Check sheet for the modelled part. Datum: model origin and axes. Units: mm. A direction names the side the tool comes from. Give positions to 0.01 mm unless a question says otherwise; leave off trailing zeros. Write each loop counter-clockwise with the first axis right and the second up, starting at its lowest first coordinate (ties: lowest second). Pieces come first, ordered by that corner, then holes. Notation, with made-up numbers: M 72.25,81.25 L 96.25,81.25 A19 ccw 96.25,108.25 Z; hole C -15,22 d9. An arc over 180 degrees is marked long. Use CSV: the item, a comma, the result in double quotes. Start each with the question number.
1. Cross-section at D-D, the plane z = -32. Enter the section's corners in (x, y).
2. Mould release check, pull along Z, two halves, no side actions. Record for faces 4 (the face through (-21, 43, -23.55)), 5 (the face through (-21, 43, 18.45)), 6 (the face through (-21.29, 35.22, -2.83)): +Z half, -Z half, draft (parallel to the pull), parting line (faces both ways), or undercut.
3. Cross-section at C-C, the plane z = 12. Enter the section's corners in (x, y).
4. Access from +Z, -Z, +X, -X, +Y, -Y to the whole of each face (thin tool, end or side, straight path). Record for faces 1 (the face through (-21, 38, 25)), 2 (the face through (0, 24, -3)), 3 (the face through (-21, 38, -30)).
5. Depth check by flat-ended pin: P1, Ø6.5, axis at x = -15, z = 26.5, coming from the +Y side; P2, Ø3, axis at x = -25.5, y = 43, coming from the -Z side; P3, Ø1, axis at x = 9, z = 27, coming from the +Y side. Enter the tip coordinate at first touch or a pass-through.
6. Cross-section at A-A, the plane x = -12. Enter the section's corners in (y, z).
7. Scan lines: line 1 (Y direction, x = 2, z = -31); line 2 (X direction, y = 44, z = -15); line 3 (Y direction, x = -25.5, z = 18.5). Record each from-to range of solid material in increasing order.
8. Cross-section at B-B, the plane y = 5.5. Enter the section's corners in (x, z), and give its area (3 significant figures).
from build123d import *

# Parameters (mm, degrees)
BOSS_EXTRUDE1_DEPTH = 21
BOSS_EXTRUDE2_DEPTH = 14


with BuildPart() as part:
    # Sketch1 → Boss-Extrude1 (new body)
    with BuildSketch(Plane(origin=(0, 0, 0), x_dir=(0, 0, -1), z_dir=(1, 0, 0))):
        with BuildLine():
            Line((-45.865633075, 14), (-45.865633075, 0))
            Line((-45.865633075, 0), (54.134366925, 0))
            Line((54.134366925, 0), (54.134366925, 14))
            Line((54.134366925, 14), (36.550387597, 38))
            Line((36.550387597, 38), (23.550387597, 38))
            Line((23.550387597, 38), (23.550387597, 48))
            Line((23.550387597, 48), (15.333333333, 48))
            ThreePointArc((15.333333333, 48), (2.550387597, 35.217054264), (-10.23255814, 48))
            Line((-10.23255814, 48), (-18.449612403, 48))
            Line((-18.449612403, 48), (-18.449612403, 38))
            Line((-18.449612403, 38), (-31.449612403, 38))
            Line((-31.449612403, 38), (-45.865633075, 14))
        make_face()
    extrude(amount=-BOSS_EXTRUDE1_DEPTH)

    # Mirror1: part across plane


with BuildPart() as part_1:
    add(part.part)
    add(part.part.mirror(Plane.ZY.offset(21)))

    # Sketch3 → Boss-Extrude2 (add)
    with BuildSketch(Plane.XZ):
        with BuildLine():
            Line((0, 27.865633075), (0, 24.200007191))
            Line((0, 24.200007191), (0, -20.725134363))
            Line((0, -20.725134363), (0, -36.134366925))
            ThreePointArc((0, -36.134366925), (22.627416998, -26.761783923), (32, -4.134366925))
            ThreePointArc((32, -4.134366925), (22.627416998, 18.493050073), (0, 27.865633075))
        make_face()
        with BuildLine():
            Line((0, -20.725134363), (0, 24.200007191))
            Line((0, 24.200007191), (0, 27.865633075))
            ThreePointArc((0, 27.865633075), (-32, -4.134366925), (0, -36.134366925))
            Line((0, -36.134366925), (0, -20.725134363))
        make_face()
    extrude(amount=-BOSS_EXTRUDE2_DEPTH)


solid = part_1.part
Worked answers:
1,outline,"M -42,0 L 15.73,0 L 15.73,14 L 0,14 L 0,38 L -42,38 Z"
2,face 4,"-Z half"
2,face 5,"+Z half"
2,face 6,"undercut"
3,outline,"M -42,0 L 27.63,0 L 27.63,14 L 0,14 L 0,48 L -42,48 Z"
4,face 1,"+Z, +X, -X, +Y"
4,face 2,"+X, +Y"
4,face 3,"-Z, +X, -X, +Y"
5,P1,"stops at y = 38"
5,P2,"stops at z = -23.55"
5,P3,"stops at y = 14"
6,outline,"M 0,-54.13 L 14,-54.13 L 38,-36.55 L 38,-23.55 L 48,-23.55 L 48,-15.33 A12.78 cw 48,10.23 L 48,18.45 L 38,18.45 L 38,31.45 L 14,45.87 L 0,45.87 Z"
7,line 1,"y = 0 to 14"
7,line 2,"x = -42 to 0"
7,line 3,"y = 0 to 38"
8,outline,"M -42,-54.13 L 0,-54.13 L 0,-36.13 A32 ccw 0,27.87 L 0,45.87 L -42,45.87 Z"
8,area,"5,810 mm^2"
